The listing builds one solid part. Answer for the finished solid, in the listing's coordinates (mm). A direction names the side the tool comes from. Give positions to 0.01 mm unless a question says otherwise; leave off trailing zeros. Loops run counter-clockwise (first coordinate to the right, second up) from the corner with the lowest first, then second, coordinate; pieces in that order, holes last. Notation, with made-up numbers: (79, 84.5) - (90, 84.5) arc R23 ccw to (90, 94.5) - close; hole circle Ø8 at (-12, -10.5). An arc over 180 degrees is marked (long way). Answer as CSV lines item,"result". Start each with the question number.
1) A cutting plane is placed at C-C (z = 10). Determine the outline of the cut face in (x, y).
2) For faces 3 (the face through (80.541, 167.367, 18.085)), 4 (the face through (80.52, 165.24, 24.16)), 5 (the face through (2, 181, 17)), determine the directions among +Z, -Z, +X, -X, +Y, -Y from which every point of the face is accessible in a straight line to the end or side of a thin tool.
3) For a pull along Z with two mould halves and no side action, classify faces 1 (the face through (1.521, 137.307, 15.564)), 2 (the face through (0, 111, 20)) as pulls with the +Z half, pulls with the -Z half, needs draft (parallel to the pull), parting line crosses it, or undercut.
4) Flat-ended cylindrical pins translate along their axes: pin 1 (10 mm diameter, centred on x = 90, z = 6, fed in from +Y); pin 2 (13 mm diameter, centred on y = 185, z = 20, fed in from +X); pin 3 (2 mm diameter, centred on x = 108.5, z = 15, fed in from +Y); pin 4 (9 mm diameter, centred on y = 25, z = 20, fed in from -X). Find the tip coordinate at first contact, or state that the pin passes through.
5) A cutting plane is placed at B-B (z = 20). Determine the outline of the cut face in (x, y), and give its area (3 significant figures).
6) Find the intervals of material crossed by line 1 along Z through (x, y) = (1.25, 25); line 2 along X through (y, z) = (188.5, 37.5); line 3 along X through (y, z) = (35.5, 21), in increasing order.
7) A cutting plane is placed at D-D (y = 112). Determine the outline of the cut face in (x, z).
8) A cutting plane is placed at A-A (y = 25). Determine the outline of the cut face in (x, z).
```python
from build123d import *

# Parameters (mm, degrees)
BOSS_EXTRUDE1_DEPTH = 40
SKETCH2_R           = 5
CUT_EXTRUDE1_DEPTH  = 40
SKETCH3_R           = 5
CUT_EXTRUDE2_DEPTH  = 40


with BuildPart() as part:
    # Sketch1 → Boss-Extrude1 (new body)
    with BuildSketch(Plane.XY):
        with BuildLine():
            Line((0, 0), (0, 225.857864376))
            ThreePointArc((0, 225.857864376), (6.173165676, 235.096659701), (17.071067812, 232.928932188))
            Line((17.071067812, 232.928932188), (141.421356237, 108.578643763))
            Line((141.421356237, 108.578643763), (139.300035894, 106.457323419))
            Line((139.300035894, 106.457323419), (20.071067812, 225.686291501))
            ThreePointArc((20.071067812, 225.686291501), (9.173165676, 227.854019014), (3, 218.615223689))
            Line((3, 218.615223689), (3, 0))
            Line((3, 0), (0, 0))
        make_face()
    extrude(amount=BOSS_EXTRUDE1_DEPTH)

    # Sketch2 → Cut-Extrude1 (cut)
    with BuildSketch(Plane(origin=(3, 0, 0), x_dir=(0, 0, -1), z_dir=(1, 0, 0))):
        with Locations(Location((-20, 185, 0), (0, 0, 90))):
            Circle(SKETCH2_R)
        with Locations(Location((-20, 25, 0), (0, 0, 90))):
            Circle(SKETCH2_R)
        with Locations(Location((-20, 135, 0), (0, 0, 90))):
            Circle(SKETCH2_R)
    extrude(amount=-CUT_EXTRUDE1_DEPTH, mode=Mode.SUBTRACT)

    # Sketch3 → Cut-Extrude2 (cut)
    with BuildSketch(Plane(origin=(125, 125, 0), x_dir=(0, 0, -1), z_dir=(0.7071067811865509, 0.7071067811865441, 0))):
        with Locations(Location((-20, 16.776695297, 0), (0, 0, 90))):
            Circle(SKETCH3_R)
        with Locations(Location((-20, 56.776695297, 0), (0, 0, 90))):
            Circle(SKETCH3_R)
    extrude(amount=-CUT_EXTRUDE2_DEPTH, mode=Mode.SUBTRACT)


solid = part.part
```
Ans:
1,outline,"(0, 0) - (3, 0) - (3, 218.62) arc R10 cw to (20.07, 225.69) - (139.3, 106.46) - (141.42, 108.58) - (17.07, 232.93) arc R10 ccw to (0, 225.86) - close"
2,face 3,"none"
2,face 4,"+Z, -Z, -Y"
2,face 5,"-X"
3,face 1,"undercut"
3,face 2,"needs draft"
4,pin 1,"y = 165"
4,pin 2,"x = 71.5"
4,pin 3,"y = 142.5"
4,pin 4,"through"
5,outline,"(0, 0) - (3, 0) - (3, 20) - (0, 20) - close; (0, 30) - (3, 30) - (3, 130) - (0, 130) - close; (0, 140) - (3, 140) - (3, 180) - (0, 180) - close; (0, 190) - (3, 190) - (3, 218.62) arc R10 cw to (20.07, 225.69) - (79.2, 166.56) - (81.32, 168.68) - (17.07, 232.93) arc R10 ccw to (0, 225.86) - close; (86.27, 159.49) - (107.48, 138.28) - (109.6, 140.4) - (88.39, 161.61) - close; (114.55, 131.21) - (139.3, 106.46) - (141.42, 108.58) - (116.67, 133.33) - close"
5,area,"1,180 mm2"
6,line 1,"0 to 15, 25 to 40"
6,line 2,"0 to 3, 57.26 to 61.5"
6,line 3,"0 to 3"
7,outline,"(0, 0) - (3, 0) - (3, 40) - (0, 40) - close; (133.76, 0) - (138, 0) - (138, 40) - (133.76, 40) - close"
8,outline,"(0, 0) - (3, 0) - (3, 15) - (0, 15) - close; (0, 25) - (3, 25) - (3, 40) - (0, 40) - close"
